The listing builds one solid part. Answer for the finished solid, in the listing's coordinates (mm). Coordinates: 2 decimals unless noted, no trailing zeros. Order: outer loops, then holes, each group sorted by start corner. A loop starts at its lowest first (then second) coordinate and runs counter-clockwise, first axis right, second up.
```python
from build123d import *

# Parameters (mm, degrees)
SKETCH1_R           = 1.625
BOSS_EXTRUDE1_DEPTH = 5


with BuildPart() as part:
    # Sketch1 → Boss-Extrude1 (new body)
    with BuildSketch(Plane(origin=(0, 0, 0), x_dir=(1, 0, 0), z_dir=(0, 1, 0))):
        with BuildLine():
            Line((15, 40), (-10, 40))
            Line((-10, 40), (-10, 3.729833462))
            ThreePointArc((-10, 3.729833462), (-31.308740902, -12.890042764), (-37.186269666, -39.266876922))
            Line((-37.186269666, -39.266876922), (-32.5, -34.266876922))
            ThreePointArc((-32.5, -34.266876922), (2.5, 0.733123078), (37.5, -34.266876922))
            Line((37.5, -34.266876922), (42.186269666, -39.266876922))
            ThreePointArc((42.186269666, -39.266876922), (36.308740902, -12.890042764), (15, 3.729833462))
            Line((15, 3.729833462), (15, 40))
        make_face()
        with Locations(Location((-4.5, 9.992204686, 0), (0, 0, 270))):
            Circle(SKETCH1_R, mode=Mode.SUBTRACT)
        with Locations(Location((-4.5, 35.992204686, 0), (0, 0, 270))):
            Circle(SKETCH1_R, mode=Mode.SUBTRACT)
        with Locations(Location((9.5, 35.992204686, 0), (0, 0, 90))):
            Circle(SKETCH1_R, mode=Mode.SUBTRACT)
        with Locations(Location((9.5, 9.992204686, 0), (0, 0, 90))):
            Circle(SKETCH1_R, mode=Mode.SUBTRACT)
    extrude(amount=BOSS_EXTRUDE1_DEPTH)


solid = part.part
```
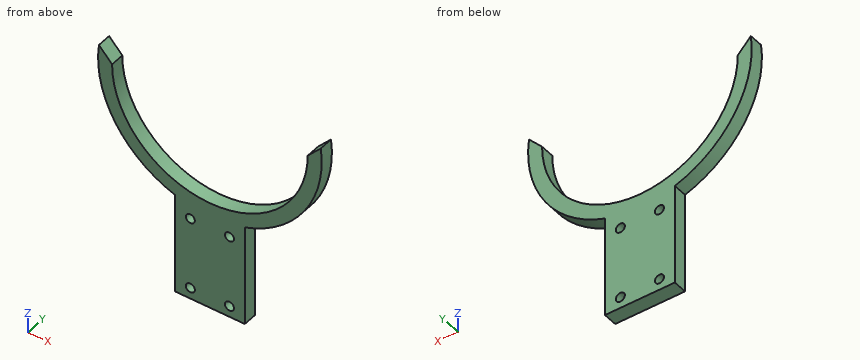
1) A cutting plane is placed at A-A, the plane x = -4.5. Write down the section's boundary in (y, z).
2) Each of these flat-tipped pins is pushed along its axis until it touches: P1, Ø1, axis at x = -25, y = 2.5, coming from the -Z side; P2, Ø2, axis at y = 1.5, z = 23, coming from the -X side; P3, Ø1, axis at x = 7, y = 4, coming from the +Z side. Where does it stop, or does it pass through?
3) Straight lines are drawn through the part: probe 1 along Z at (x, y) = (9.5, 2.6); probe 2 along X at (y, z) = (0.7, -8.5); probe 3 along X at (y, z) = (0.25, 27). For each, find the intervals that lie inside material, in ascending order.
4) A cutting plane is placed at B-B, the plane z = 25.5. Write down the section's boundary in (x, y), plus the area to 3 significant figures.
5) A cutting plane is placed at D-D, the plane x = -22. Write down the section's boundary in (y, z), plus the area to 3 significant figures.
6) A cutting plane is placed at C-C, the plane y = 1.3. Write down the section's boundary in (x, z) (3 decimals), plus the area to 3 significant figures.
Working result:
1. outline: (0, -40) - (5, -40) - (5, -37.62) - (0, -37.62) - close; (0, -34.37) - (5, -34.37) - (5, -11.62) - (0, -11.62) - close; (0, -8.37) - (5, -8.37) - (5, -0.03) - (0, -0.03) - close
2. P1: stops at z = 4.75
2. P2: stops at x = -36.16
2. P3: stops at z = -0.37
3. probe 1: z = -40 to -37.62, -34.37 to -11.62, -8.37 to -0.03
3. probe 2: x = -10 to -5.14, -3.86 to 8.86, 10.14 to 15
3. probe 3: x = -36.83 to -31.74, 36.74 to 41.83
4. outline: (-36.53, 0) - (-31.38, 0) - (-31.38, 5) - (-36.53, 5) - close; (36.38, 0) - (41.53, 0) - (41.53, 5) - (36.38, 5) - close
4. area: 51.4 mm2
5. outline: (0, 2.65) - (5, 2.65) - (5, 9.27) - (0, 9.27) - close
5. area: 33.1 mm2
6. outline: (-37.186, 39.267) arc R40 ccw to (-10, -3.73) - (-10, -40) - (15, -40) - (15, -3.73) arc R40 ccw to (42.186, 39.267) - (37.5, 34.267) arc R35 cw to (-32.5, 34.267) - close; hole circle Ø3.25 at (-4.5, -35.992); hole circle Ø3.25 at (-4.5, -9.992); hole circle Ø3.25 at (9.5, -35.992); hole circle Ø3.25 at (9.5, -9.992)
6. area: 1,450 mm2
